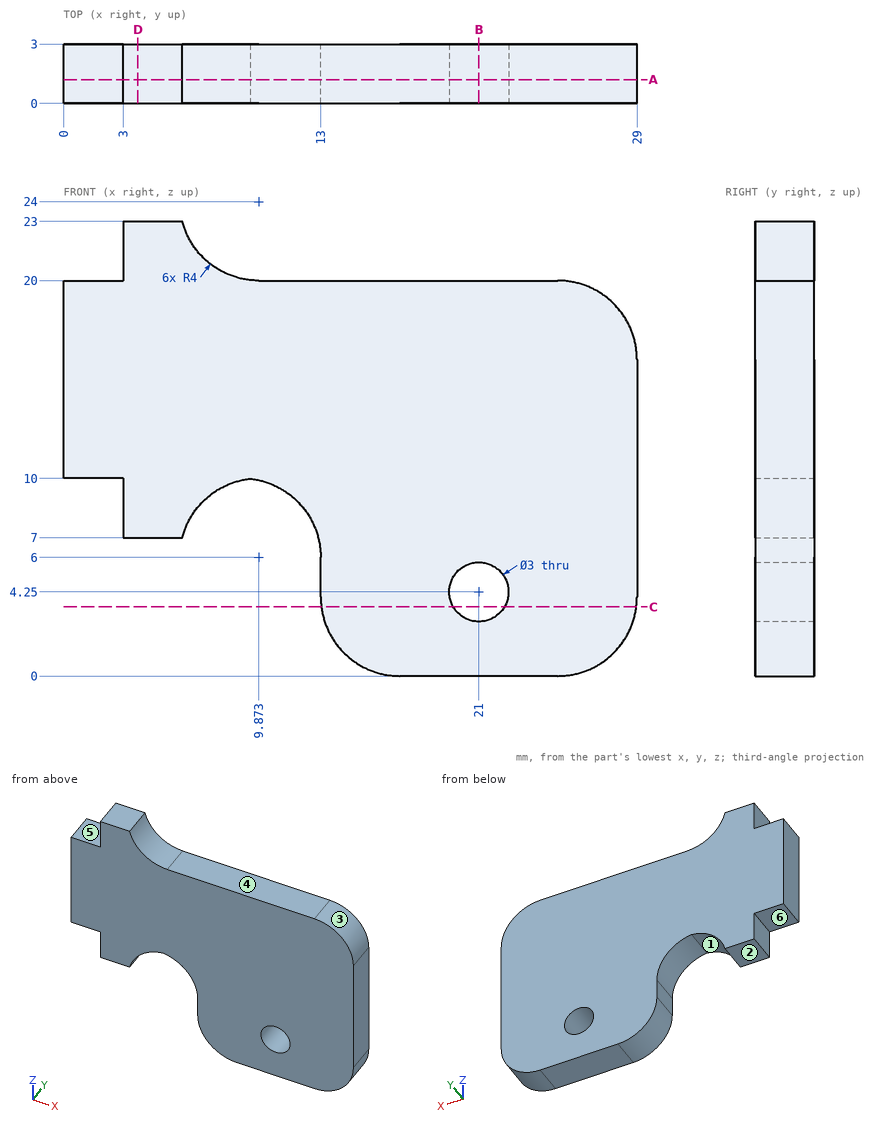
Geometry check sheet. Reference: drawing and pictorial views, mm from the part's lowest x, y, z. A direction names the side the tool comes from. Give positions to 0.01 mm unless a question says otherwise; leave off trailing zeros. Write each loop counter-clockwise with the first axis right and the second up, starting at its lowest first coordinate (ties: lowest second). Pieces come first, ordered by that corner, then holes. Notation, with made-up numbers: M 22.5,5 L 38.5,5 A24 cw 38.5,22 Z; hole C -33.5,85.5 d11. An arc over 180 degrees is marked long. Put each result on its own line as item: value. Start each with the question number.
1. Section check B-B (x = 21). Record the cut outline in (y, z).
2. Section check C-C (z = 3.5). Record the cut outline in (x, y).
3. Set-up check for the marked faces 4, 5 and 6: record each of +Z, -Z, +X, -X, +Y, -Y from which the full face is reachable in a straight line by a thin tool's end or side.
4. Scan lines: line 1 along X through (y, z) = (1.9, 4.25); line 2 along X through (y, z) = (1.95, 3.75); line 3 along Z through (x, y) = (27.25, 2.55). Record each from-to range of solid material in increasing order. Write a range as [from, to].
5. Section check A-A (y = 1.2). Record the cut outline in (x, z).
6. Draft check along X on the marked faces 1, 2 and 3. Enter one of: +X half, -X half, draft (parallel to the pull), parting line (faces both ways), or undercut.
7. Go/stop test with flat-tipped pins: pin 1 Ø0.9 at (x, y) = (1, 2) entering from +Z; pin 2 Ø1.6 at (y, z) = (1, 5.5) entering from -X; pin 3 Ø1.5 at (x, y) = (1.5, 1) entering from -Z. Record where each tip stops, or that it passes through.
8. Section check D-D (x = 3.75). Record the cut outline in (y, z), and give its area (3 significant figures).
Answer list:
1. outline: M 0,0 L 3,0 L 3,2.75 L 0,2.75 Z; M 0,5.75 L 3,5.75 L 3,20 L 0,20 Z
2. outline: M 13.03,0 L 19.7,0 L 19.7,3 L 13.03,3 Z; M 22.3,0 L 28.97,0 L 28.97,3 L 22.3,3 Z
3. face 4: +Z, +X, +Y, -Y
3. face 5: +Z, -X, +Y, -Y
3. face 6: -Z, -X, +Y, -Y
4. line 1: [13, 19.5], [22.5, 29]
4. line 2: [13.01, 19.59], [22.41, 28.99]
4. line 3: [0.69, 19.31]
5. outline: M 0,10 L 3,10 L 3,7 L 6,7 A4 cw 9.44,9.98 A4 cw 13,6 L 13,4 A4 ccw 17,0 L 25,0 A4 ccw 29,4 L 29,16 A4 ccw 25,20 L 9.87,20 A4 cw 6,23 L 3,23 L 3,20 L 0,20 Z; hole C 21,4.25 d3
6. face 1: undercut
6. face 2: draft
6. face 3: +X half
7. pin 1: z = 20
7. pin 2: x = 12.99
7. pin 3: z = 10
8. outline: M 0,7 L 3,7 L 3,23 L 0,23 Z
8. area: 48.0 mm2
